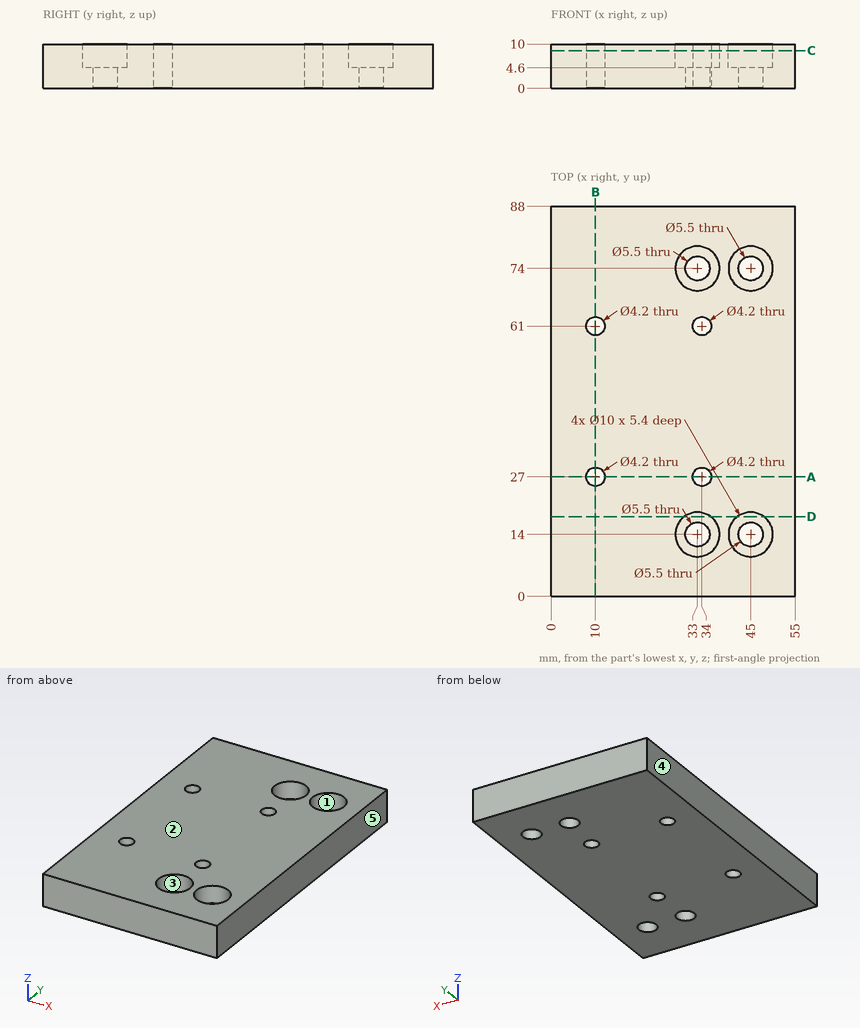
Answer from the drawing. Dimensions are ordinates in mm from the lowest x, y and z of the part. A direction names the side the tool comes from. Give positions to 0.01 mm unless a question says otherwise; leave off trailing zeros. Loops run counter-clockwise (first coordinate to the right, second up) from the corner with the lowest first, then second, coordinate; pieces in that order, holes last. Notation, with made-up numbers: (-24, 0.5) -> (11, 0.5) arc R29 cw to (11, 38.5) -> close; hole circle Ø7 at (76.5, -33.5). An arc over 180 degrees is marked (long way). Use a Markdown table: item, result.
Q1. Find the intervals of material crossed by line 1 along Y through (x, z) = (45, 2.1); line 2 along X through (y, z) = (74, 2.75); line 3 along Y through (x, z) = (45, 8.4), in increasing order.
Solved:
| item | result |
|---|---|
| line 1 | y = 0 to 11.25, 16.75 to 71.25, 76.75 to 88 |
| line 2 | x = 0 to 30.25, 35.75 to 42.25, 47.75 to 55 |
| line 3 | y = 0 to 9, 19 to 69, 79 to 88 |
Q2. A tool of negligible diameter and unlimited length cuts with its end or side. For the marked faces 1 and 2, from which of +Z, -Z, +X, -X, +Y, -Y can it reach the whole face along a straight path? Write none if from no direction.
Solved:
| item | result |
|---|---|
| face 1 | +Z |
| face 2 | +Z, +X, -X, +Y, -Y |
Q3. Section D-D, the plane y = 18 is taken. Determine the outline of the cut face in (x, z).
Solved:
| item | result |
|---|---|
| outline | (0, 0) -> (55, 0) -> (55, 10) -> (48, 10) -> (48, 4.6) -> (42, 4.6) -> (42, 10) -> (36, 10) -> (36, 4.6) -> (30, 4.6) -> (30, 10) -> (0, 10) -> close |
Q4. Determine the mould class of the marked faces 3, 4 and 5 for opening direction X: pulls with the +X half, pulls with the -X half, needs draft (parallel to the pull), parting line crosses it, or undercut.
Solved:
| item | result |
|---|---|
| face 3 | undercut |
| face 4 | pulls with the -X half |
| face 5 | pulls with the +X half |
Q5. Each of these flat-tipped pins is pushed along its axis until it touches: pin 1 (11 mm diameter, centred on x = 43.5, y = 13.5, fed in from +Z); pin 2 (3 mm diameter, centred on x = 31.5, y = 12.5, fed in from +Z). Where does it stop, or does it pass through?
Solved:
| item | result |
|---|---|
| pin 1 | stops at z = 10 |
| pin 2 | stops at z = 4.6 |
Q6. Section B-B, the plane x = 10 is taken. Determine the outline of the cut face in (y, z), then the cut area to 3 significant figures.
Solved:
| item | result |
|---|---|
| outline | (0, 0) -> (24.9, 0) -> (24.9, 10) -> (0, 10) -> close; (29.1, 0) -> (58.9, 0) -> (58.9, 10) -> (29.1, 10) -> close; (63.1, 0) -> (88, 0) -> (88, 10) -> (63.1, 10) -> close |
| area | 796 mm^2 |
Q7. Section A-A, the plane y = 27 is taken. Determine the outline of the cut face in (x, z).
Solved:
| item | result |
|---|---|
| outline | (0, 0) -> (7.9, 0) -> (7.9, 10) -> (0, 10) -> close; (12.1, 0) -> (31.9, 0) -> (31.9, 10) -> (12.1, 10) -> close; (36.1, 0) -> (55, 0) -> (55, 10) -> (36.1, 10) -> close |
Q8. Section C-C, the plane z = 8.5 is taken. Count the separate pieces of the cut face and the enclosed holes in it, then the cut area to 3 significant figures.
Solved:
| item | result |
|---|---|
| separate pieces | 1 |
| enclosed holes | 8 |
| area | 4,470 mm^2 |
